```python
from build123d import *

# Parameters (mm, degrees)
SKETCH1_R           = 5
SKETCH1_R_2         = 1.7
SKETCH1_W           = 10
SKETCH1_H           = 15
BOSS_EXTRUDE1_DEPTH = 2
SKETCH2_W           = 45
SKETCH2_H           = 4.5
BOSS_EXTRUDE2_DEPTH = 6.85
BOSS_EXTRUDE3_START = 3.5
SKETCH3_W           = 45
SKETCH3_H           = 4.5
BOSS_EXTRUDE3_DEPTH = 3.5
CUT_EXTRUDE1_DEPTH  = 2.5
CUT_EXTRUDE2_REACH  = 53.154
SKETCH4_R           = 1.2
CUT_EXTRUDE3_DEPTH  = 1
CUT_EXTRUDE4_REACH  = 53.154
SKETCH6_R           = 1.7


with BuildPart() as part:
    # Sketch1 → Boss-Extrude1 (new body)
    # profile 1 of 5: a face of its own
    with BuildSketch(Plane(origin=(0, 0, 0), x_dir=(1, 0, 0), z_dir=(0, 1, 0))):
        Circle(SKETCH1_R)
        with Locations(Location((0, 0, 0), (0, 0, 270))):
            Circle(SKETCH1_R_2, mode=Mode.SUBTRACT)
    # profile 2 of 5: a face of its own
    with BuildSketch(Plane(origin=(0, 0, 0), x_dir=(1, 0, 0), z_dir=(0, 1, 0))):
        with BuildLine():
            ThreePointArc((5, 0), (-3.292912646, -3.762542532), (-0.662690524, 4.955889554))
            Line((-0.662690524, 4.955889554), (-27.725, 1.337177748))
            Line((-27.725, 1.337177748), (-27.725, -15))
            Line((-27.725, -15), (-12.725, -15))
            Line((-12.725, -15), (39.55, -15))
            Line((39.55, -15), (39.55, 0))
            ThreePointArc((39.55, 0), (31.014466094, -3.535533906), (34.55, 5))
            Line((34.55, 5), (0, 5))
            ThreePointArc((0, 5), (3.535533906, 3.535533906), (5, 0))
        make_face()
    # profile 3 of 5: a face of its own
    with BuildSketch(Plane(origin=(0, 0, 0), x_dir=(1, 0, 0), z_dir=(0, 1, 0))):
        with Locations((34.55, 0)):
            Circle(SKETCH1_R)
        with Locations(Location((34.55, 0, 0), (0, 0, 270))):
            Circle(SKETCH1_R_2, mode=Mode.SUBTRACT)
    # profile 4 of 5: a face of its own
    with BuildSketch(Plane(origin=(0, 0, 0), x_dir=(1, 0, 0), z_dir=(0, 1, 0))):
        with Locations((-32.725, -22.5)):
            Rectangle(SKETCH1_W, SKETCH1_H)
    # profile 5 of 5: a face of its own
    with BuildSketch(Plane(origin=(0, 0, 0), x_dir=(1, 0, 0), z_dir=(0, 1, 0))):
        Polygon((-12.725, -15), (-27.725, -15), (-27.725, -30), align=None)
    extrude(amount=BOSS_EXTRUDE1_DEPTH)

    # Sketch2 → Boss-Extrude2 (add)
    with BuildSketch(Plane.XZ):
        with Locations((17.05, 12.75)):
            Rectangle(SKETCH2_W, SKETCH2_H)
    extrude(amount=BOSS_EXTRUDE2_DEPTH)

    # Sketch3 → Boss-Extrude3 (add)
    # profile 1 of 4: a face of its own
    with BuildSketch(Plane.XZ.offset(6.85).offset(BOSS_EXTRUDE3_START)):
        with BuildLine():
            Line((0, -5), (34.55, -5))
            ThreePointArc((34.55, -5), (38.085533906, -3.535533906), (39.55, 0))
            Line((39.55, 0), (39.55, 10.5))
            Line((39.55, 10.5), (-5.45, 10.5))
            Line((-5.45, 10.5), (-5.45, -4.315741183))
            Line((-5.45, -4.315741183), (-0.662690524, -4.955889554))
            ThreePointArc((-0.662690524, -4.955889554), (-0.332078478, -4.988960201), (0, -5))
        make_face()
        Polygon((37.898631561, 0), (36.224315781, 2.9), (32.875684219, 2.9), (31.201368439, 0), (32.875684219, -2.9), (36.224315781, -2.9), align=None, mode=Mode.SUBTRACT)
        Polygon((3.348631561, 0), (1.674315781, 2.9), (-1.674315781, 2.9), (-3.348631561, 0), (-1.674315781, -2.9), (1.674315781, -2.9), align=None, mode=Mode.SUBTRACT)
    # profile 2 of 4: a face of its own
    with BuildSketch(Plane.XZ.offset(6.85).offset(BOSS_EXTRUDE3_START)):
        Polygon((1.674315781, -2.9), (3.348631561, 0), (1.674315781, 2.9), (-1.674315781, 2.9), (-3.348631561, 0), (-1.674315781, -2.9), align=None)
    # profile 3 of 4: a face of its own
    with BuildSketch(Plane.XZ.offset(6.85).offset(BOSS_EXTRUDE3_START)):
        Polygon((36.224315781, -2.9), (37.898631561, 0), (36.224315781, 2.9), (32.875684219, 2.9), (31.201368439, 0), (32.875684219, -2.9), align=None)
    # profile 4 of 4: a face of its own
    with BuildSketch(Plane.XZ.offset(6.85).offset(BOSS_EXTRUDE3_START)):
        with Locations((17.05, 12.75)):
            Rectangle(SKETCH3_W, SKETCH3_H)
    extrude(amount=-BOSS_EXTRUDE3_DEPTH)

    # Sketch3_3 → Cut-Extrude1 (cut)
    with BuildSketch(Plane.XZ.offset(6.85)):
        Polygon((36.224315781, -2.9), (37.898631561, 0), (36.224315781, 2.9), (32.875684219, 2.9), (31.201368439, 0), (32.875684219, -2.9), align=None)
        Polygon((1.674315781, -2.9), (3.348631561, 0), (1.674315781, 2.9), (-1.674315781, 2.9), (-3.348631561, 0), (-1.674315781, -2.9), align=None)
    extrude(amount=CUT_EXTRUDE1_DEPTH, mode=Mode.SUBTRACT)

    # Sketch4 → Cut-Extrude2 (cut, up to next)
    with BuildSketch(Plane(origin=(0, 2, 0), x_dir=(1, 0, 0), z_dir=(0, 1, 0)), mode=Mode.PRIVATE) as cut_extrude2_sk1:
        with Locations(Location((-33.225, -20.6, 0), (0, 0, 270))):
            Circle(SKETCH4_R)
    cut_extrude2_tool1 = extrude(cut_extrude2_sk1.sketch, amount=-CUT_EXTRUDE2_REACH, mode=Mode.PRIVATE) & part.part
    # Sketch4 → Cut-Extrude2 (cut, up to next)
    with BuildSketch(Plane(origin=(0, 2, 0), x_dir=(1, 0, 0), z_dir=(0, 1, 0)), mode=Mode.PRIVATE) as cut_extrude2_sk2:
        with Locations(Location((-33.225, -27, 0), (0, 0, 270))):
            Circle(SKETCH4_R)
    cut_extrude2_tool2 = extrude(cut_extrude2_sk2.sketch, amount=-CUT_EXTRUDE2_REACH, mode=Mode.PRIVATE) & part.part
    add(cut_extrude2_tool1.solids().sort_by_distance((-33.225, 2, 20.6))[0], mode=Mode.SUBTRACT)
    add(cut_extrude2_tool2.solids().sort_by_distance((-33.225, 2, 27))[0], mode=Mode.SUBTRACT)

    # Sketch5 → Cut-Extrude3 (cut)
    with BuildSketch(Plane.XZ):
        Polygon((-32.012564435, 22.7), (-34.437435565, 22.7), (-35.649871131, 20.6), (-34.437435565, 18.5), (-32.012564435, 18.5), (-30.800128869, 20.6), align=None)
        Polygon((-32.012564435, 29.1), (-34.437435565, 29.1), (-35.649871131, 27), (-34.437435565, 24.9), (-32.012564435, 24.9), (-30.800128869, 27), align=None)
    extrude(amount=-CUT_EXTRUDE3_DEPTH, mode=Mode.SUBTRACT)

    # Sketch6 → Cut-Extrude4 (cut, up to next)
    with BuildSketch(Plane.XZ.offset(10.35), mode=Mode.PRIVATE) as cut_extrude4_sk1:
        with Locations(Location((0, 0, 0), (0, 0, 90))):
            Circle(SKETCH6_R)
    cut_extrude4_tool1 = extrude(cut_extrude4_sk1.sketch, amount=-CUT_EXTRUDE4_REACH, mode=Mode.PRIVATE) & part.part
    # Sketch6 → Cut-Extrude4 (cut, up to next)
    with BuildSketch(Plane.XZ.offset(10.35), mode=Mode.PRIVATE) as cut_extrude4_sk2:
        with Locations(Location((34.55, 0, 0), (0, 0, 90))):
            Circle(SKETCH6_R)
    cut_extrude4_tool2 = extrude(cut_extrude4_sk2.sketch, amount=-CUT_EXTRUDE4_REACH, mode=Mode.PRIVATE) & part.part
    add(cut_extrude4_tool1.solids().sort_by_distance((0, -10.35, 0))[0], mode=Mode.SUBTRACT)
    add(cut_extrude4_tool2.solids().sort_by_distance((34.55, -10.35, 0))[0], mode=Mode.SUBTRACT)


solid = part.part
```
Can you work these out from the model? Positions are in its coordinate system, mm. A direction names the side the tool comes from. Round coordinates to 2 decimals unless told otherwise and drop trailing zeros. Loops run counter-clockwise (first coordinate to the right, second up) from the corner with the lowest first, then second, coordinate; pieces in that order, holes last. Notation, with made-up numbers: M -36,10.5 L -10,10.5 A31 cw -10,40.5 Z; hole C 31.25,-1 d7. An arc over 180 degrees is marked long. Answer as a JSON object with one key per item and string values. Group by question number.
Q1. Imagine slicing it at A-A, the plane z = 4. Please give me the cut outline in (x, y) (3 decimals).
Q2. Please list where these lines run through material, in increasing order: L1, parallel to X at y = -9.75, z = 0; L2, parallel to X at y = 1, z = 0 (3 decimals); L3, parallel to Z at x = 1.5, y = -7.25.
Q3. We'd pull the mould along X, two halves only. Please class faces 1 (the flat face through (36, -9.35, 1.3)), 2 (the flat face through (-33, 1, 30)), 3 (the cylindrical face through (38.12, 0.99, -3.5)), 4 (the flat face through (-27.725, 1, 7)): +X half, -X half, draft (parallel to the pull), parting line (faces both ways), or undercut.
Q4. Imagine slicing it at C-C, the plane z = 12.5. Please give me the cut outline in (x, y) (3 decimals).
Q5. On a 3-axis mill with a long thin cutter (end or side, diameter ignored), from which of +Z, -Z, +X, -X, +Y, -Y can I reach the whole of each face in a straight line? I mean faces 5 (the flat face through (-33, 1, 15)), 6 (the flat face through (13, -4, 15)), 7 (the flat face through (-32, 1, 28)), 8 (the flat face through (35, -8, 2.9)). Say none if no direction works.
Q6. Imagine slicing it at B-B, the plane x = 14. Please give me the cut outline in (y, z), then the cut area to 3 significant figures.
Q7. Will these pins go through, and if not, where does the flat tip stop? pin 1 (0.8 mm diameter, centred on x = 0.5, y = -8.5, fed in from +Z); pin 2 (1.5 mm diameter, centred on y = -7, z = 13.5, fed in from -X); pin 3 (5 mm diameter, centred on y = -1, z = 7.5, fed in from +X); pin 4 (2 mm diameter, centred on x = 0, z = 0, fed in from -Y).
Q8. Imagine slicing it at D-D, the plane y = -1.5. Please give me the cut outline in (x, z), then the cut area to 4 significant figures.
Findings:
{
 "1": {"outline": "M -27.725,0 L 39.55,0 L 39.55,2 L -27.725,2 Z; M -5.45,-10.35 L 39.55,-10.35 L 39.55,-6.85 L -5.45,-6.85 Z"},
 "2": {"L1": "x = -5.45 to -1.7, 1.7 to 32.85, 36.25 to 39.55", "L2": "x = -27.725 to -1.7, 1.7 to 32.85, 36.25 to 39.55", "L3": "z = -5 to -2.9, 2.9 to 15"},
 "3": {"face 1": "undercut", "face 2": "draft", "face 3": "+X half", "face 4": "-X half"},
 "4": {"outline": "M -27.725,0 L -5.45,0 L -5.45,-10.35 L 39.55,-10.35 L 39.55,2 L -27.725,2 Z"},
 "5": {"face 5": "-Z, -X, +Y, -Y", "face 6": "+Z, +X, +Y, -Y", "face 7": "-Y", "face 8": "none"},
 "6": {"outline": "M -10.35,-5 L -6.85,-5 L -6.85,10.5 L 0,10.5 L 0,-5 L 2,-5 L 2,15 L -10.35,15 Z", "area": "141 mm2"},
 "7": {"pin 1": "stops at z = 15", "pin 2": "stops at x = -5.45", "pin 3": "stops at x = 39.55", "pin 4": "passes through"},
 "8": {"outline": "M -5.45,10.5 L 39.55,10.5 L 39.55,15 L -5.45,15 Z", "area": "202.5 mm2"}
}
